Geometry: final body of the model. Coordinates: model frame, mm. Face numbers are marked on the shaded views. A direction names the side the tool comes from. Coordinates: 2 decimals unless noted, no trailing zeros. Write each loop counter-clockwise with the first axis right and the second up, starting at its lowest first coordinate (ties: lowest second). Pieces come first, ordered by that corner, then holes.
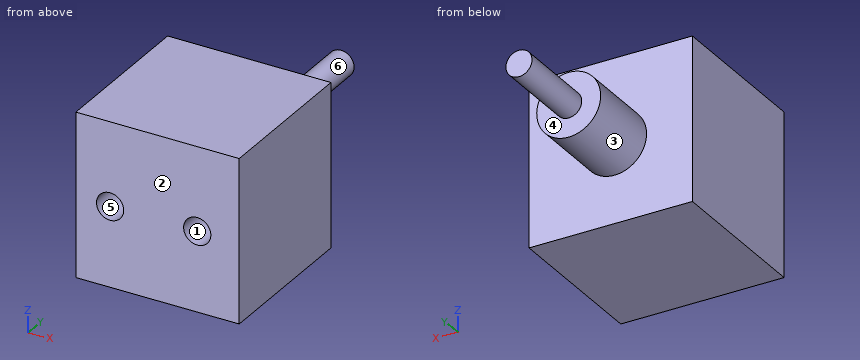
from build123d import *

# Parameters (mm, degrees)
SKETCH_1_W          = 30
SKETCH_1_H          = 30
EXTRUDE_283_DEPTH   = 28.77
SKETCH_2_R          = 5.875
EXTRUDE_2_DEPTH     = 14.4
SKETCH_4_R          = 2.4
EXTRUDE_3_DEPTH     = 15.6
SKETCH_5_R          = 2.5
CUT_EXTRUDE_2_DEPTH = 15


with BuildPart() as part:
    # Эскиз1 → Extrude 283 (new body)
    with BuildSketch(Plane(origin=(0, 0, 0), x_dir=(1, 0, 0), z_dir=(0, 1, 0))):
        with Locations((0.713469456, -0.356734728)):
            Rectangle(SKETCH_1_W, SKETCH_1_H)
    extrude(amount=EXTRUDE_283_DEPTH)

    # Эскиз2 → Бобышка-Вытянуть2 (add)
    with BuildSketch(Plane(origin=(0, 28.77, 0), x_dir=(1, 0, 0), z_dir=(0, 1, 0))):
        with Locations(Location((0, 0, 0), (0, 0, 270))):
            Circle(SKETCH_2_R)
    extrude(amount=EXTRUDE_2_DEPTH)

    # Эскиз4 → Бобышка-Вытянуть3 (add)
    with BuildSketch(Plane(origin=(0, 43.17, 0), x_dir=(1, 0, 0), z_dir=(0, 1, 0))):
        with Locations(Location((0, 0, 0), (0, 0, 270))):
            Circle(SKETCH_4_R)
    extrude(amount=EXTRUDE_3_DEPTH)

    # Эскиз5 → Вырез-Вытянуть2 (cut)
    with BuildSketch(Plane.XZ):
        with Locations(Location((8, 0, 0), (0, 0, 270))):
            Circle(SKETCH_5_R)
        with Locations(Location((-8, 0, 0), (0, 0, 90))):
            Circle(SKETCH_5_R)
    extrude(amount=-CUT_EXTRUDE_2_DEPTH, mode=Mode.SUBTRACT)


solid = part.part
Item 1: Pin query (flat end, axial travel): pin 1 (5.5 mm diameter, centred on x = 8, z = -0.5, fed in from -Y); pin 2 (6 mm diameter, centred on x = -8, z = 0, fed in from +Y); pin 3 (10 mm diameter, centred on y = 49.5, z = 3, fed in from -X); pin 4 (3 mm diameter, centred on x = 10.5, z = -3, fed in from +Y). Return the tip coordinate at first contact, or that it passes through.
Derived:
pin 1: stops at y = 0
pin 2: stops at y = 43.17
pin 3: stops at x = -2.4
pin 4: stops at y = 28.77
Item 2: Section B-B, the plane z = 0. Output: boundary loops of the cut face in (x, y) (3 decimals).
Derived:
outline: (-14.287, 0) - (-10.5, 0) - (-10.5, 15) - (-5.5, 15) - (-5.5, 0) - (5.5, 0) - (5.5, 15) - (10.5, 15) - (10.5, 0) - (15.713, 0) - (15.713, 28.77) - (5.875, 28.77) - (5.875, 43.17) - (2.4, 43.17) - (2.4, 58.77) - (-2.4, 58.77) - (-2.4, 43.17) - (-5.875, 43.17) - (-5.875, 28.77) - (-14.287, 28.77) - close
Item 3: Section A-A, the plane x = -9.5. Output: boundary loops of the cut face in (y, z), plus the area to 3 significant figures.
Derived:
outline: (0, -14.64) - (28.77, -14.64) - (28.77, 15.36) - (0, 15.36) - (0, 2) - (15, 2) - (15, -2) - (0, -2) - close
area: 803 mm2
Item 4: Section D-D, the plane x = 0. Output: boundary loops of the cut face in (y, z) (3 decimals).
Derived:
outline: (0, -14.643) - (28.77, -14.643) - (28.77, -5.875) - (43.17, -5.875) - (43.17, -2.4) - (58.77, -2.4) - (58.77, 2.4) - (43.17, 2.4) - (43.17, 5.875) - (28.77, 5.875) - (28.77, 15.357) - (0, 15.357) - close
Item 5: Pull-direction query (X, two-part tool) for the marked faces 4, 5 and 6; classes: released by +X, released by -X, zero draft, split by the parting line, or undercut.
Derived:
face 4: zero draft
face 5: undercut
face 6: split by the parting line
Item 6: Material intervals for probe 1 along X at (y, z) = (5.5, 0); probe 2 along Y at (x, z) = (-11, 7); probe 3 along Y at (x, z) = (-6.75, 1.5), sorted ascending.
Derived:
probe 1: x = -14.29 to -10.5, -5.5 to 5.5, 10.5 to 15.71
probe 2: y = 0 to 28.77
probe 3: y = 15 to 28.77
Item 7: Set-up query: the marked faces 1, 2 and 3. Return all of +Z, -Z, +X, -X, +Y, -Y with unobstructed straight access to the full face (end or side cutting, diameter ignored); none if empty.
Derived:
face 1: -Y
face 2: +Z, -Z, +X, -X, -Y
face 3: +Y
Item 8: Section C-C, the plane y = 41. Output: boundary loops of the cut face in (x, z) (3 decimals).
Derived:
outline: circle Ø11.75 at (0, 0)
